from build123d import *

# Parameters (mm, degrees)
F1_DEPTH   = 12.7
F2_SIZE2   = 17.5976362049
F2_SIZE    = 10.16
F2_2_SIZE2 = 17.5976362049
F2_2_SIZE  = 10.16
F3_SIZE2   = 10.16
F3_SIZE    = 17.5976362049
F3_2_SIZE2 = 10.16
F3_2_SIZE  = 17.5976362049
F4_SIZE2   = 10.16
F4_SIZE    = 17.5976362049


with BuildPart() as f1:
    # F0 (on Top) → F1 (new body)
    with BuildSketch(Plane.XY):
        Polygon((12.7, 38.1), (-12.7, 38.1), (-12.7, 12.7), (-38.1, 12.7), (-38.1, -12.7), (-12.7, -12.7), (-12.7, -38.1), (12.7, -38.1), (12.7, -12.7), (38.1, -12.7), (38.1, 12.7), (12.7, 12.7), align=None)
    extrude(amount=F1_DEPTH)

    # F2
    f2_edges = [f1.edges().sort_by_distance(p)[0] for p in [
        (-12.7, -25.4, 0),
    ]]
    f2_side = f1.faces().sort_by_distance((-12.7, -25.4, 6.35))[0]
    chamfer(f2_edges, length=F2_SIZE, length2=F2_SIZE2, reference=f2_side)

    # F2#2
    f2_2_edges = [f1.edges().sort_by_distance(p)[0] for p in [
        (12.7, -25.4, 12.7),
    ]]
    f2_2_side = f1.faces().sort_by_distance((12.7, -25.4, 6.35))[0]
    chamfer(f2_2_edges, length=F2_2_SIZE, length2=F2_2_SIZE2, reference=f2_2_side)

    # F3
    f3_edges = [f1.edges().sort_by_distance(p)[0] for p in [
        (-25.4, 12.7, 0),
        (12.7, 25.4, 0),
        (25.4, -12.7, 0),
    ]]
    f3_side = f1.faces().sort_by_distance((0.627515, 4.085652, 0))[0]
    chamfer(f3_edges, length=F3_SIZE, length2=F3_SIZE2, reference=f3_side)

    # F3#2
    f3_2_edges = [f1.edges().sort_by_distance(p)[0] for p in [
        (-25.4, -12.7, 12.7),
    ]]
    f3_2_side = f1.faces().sort_by_distance((-0.627515, 4.085652, 12.7))[0]
    chamfer(f3_2_edges, length=F3_2_SIZE, length2=F3_2_SIZE2, reference=f3_2_side)

    # F4
    f4_edges = [f1.edges().sort_by_distance(p)[0] for p in [
        (-12.7, 25.4, 12.7),
        (25.4, 12.7, 12.7),
    ]]
    f4_side = f1.faces().sort_by_distance((4.121012, 5.616612, 12.7))[0]
    chamfer(f4_edges, length=F4_SIZE, length2=F4_SIZE2, reference=f4_side)


solid = f1.part
Geometry check sheet. Reference: the model listing, model coordinates, mm. A direction names the side the tool comes from. Give positions to 0.01 mm unless a question says otherwise; leave off trailing zeros. Write each loop counter-clockwise with the first axis right and the second up, starting at its lowest first coordinate (ties: lowest second). Pieces come first, ordered by that corner, then holes. Notation, with made-up numbers: M 9.5,-7 L 37.5,-7 A6 ccw 37.5,4 Z; hole C -20.5,-30 d2. An arc over 180 degrees is marked long. Answer as CSV lines item,"result". Start each with the question number.
Q1. Section check D-D, the plane x = -3. Record the cut outline in (y, z), then the cut area to 3 significant figures.
Q2. Tool access check on faces 1 (the face through (-12.7, 17, 1)), 2 (the face through (-22.82, 4.02, 5.15)), 3 (the face through (17, 12.7, 1)), 4 (the face through (3.78, -23.36, 7.69)). Record the directions out of +Z, -Z, +X, -X, +Y, -Y that give a thin tool (end or side, any length) a straight path to the whole face; none if there is none.
Q3. Material ranges on L1, parallel to Y at x = -9.5, z = 2.25; L2, parallel to Z at x = 12, y = -11; L3, parallel to Z at x = -11, y = -10.5, recorded low to high.
Q4. Go/stop test with flat-tipped pins: pin 1 (3 mm diameter, centred on y = -8.5, z = 1.5, fed in from +X); pin 2 (1 mm diameter, centred on x = -15.5, z = 9.5, fed in from +Y); pin 3 (1.3 mm diameter, centred on x = 13, z = 11, fed in from -Y); pin 4 (4 mm diameter, centred on y = -10.5, z = 4.5, fed in from -X). Record where each tip stops, or that it passes through.
Q5. Release check for a two-part mould opening along Z. For faces 5 (the face through (0, 3, 12.7)), 6 (the face through (-16, 12.7, 11)), 7 (the face through (4.02, 22.82, 5.15)) record: pulls with the +Z half, pulls with the -Z half, needs draft (parallel to the pull), parting line crosses it, or undercut.
Q6. Section check C-C, the plane z = 4.75. Record the cut outline in (x, y).
Q7. Section check A-A, the plane x = -18. Record the cut outline in (y, z), then the cut area to 3 significant figures.
Geometry says:
1,outline,"M -38.1,4.56 L -9.2,4.56 L -12.7,2.54 L -12.7,0 L 12.7,0 L 12.7,1.1 L 38.1,1.1 L 38.1,8.14 L 9.2,8.14 L 12.7,10.16 L 12.7,12.7 L -12.7,12.7 L -12.7,11.6 L -38.1,11.6 Z"
1,area,"673 mm^2"
2,face 1,"-Z, -X, +Y"
2,face 2,"-X, +Y"
2,face 3,"-Z, +X, +Y"
2,face 4,"+X, -Y"
3,L1,"-12.7 to 38.1"
3,L2,"0 to 2.94, 9.18 to 12.7"
3,L3,"0 to 3.81, 9.18 to 12.7"
4,pin 1,"x = 12.7"
4,pin 2,"y = 12.42"
4,pin 3,"y = -12.7"
4,pin 4,"x = -38.1"
5,face 5,"pulls with the +Z half"
5,face 6,"needs draft"
5,face 7,"undercut"
6,outline,"M -38.1,-8.87 L -3.33,-8.87 L -3.33,-38.1 L 8.87,-38.1 L 8.87,-3.33 L 38.1,-3.33 L 38.1,8.87 L 3.33,8.87 L 3.33,38.1 L -8.87,38.1 L -8.87,3.33 L -38.1,3.33 Z"
7,outline,"M -12.7,0 L -4.9,0 L 12.7,10.16 L 12.7,12.7 L 4.9,12.7 L -12.7,2.54 Z"
7,area,"144 mm^2"
